Read the model definition and answer for the solid it produces. Units are mm, in the model's axes. A direction names the side the tool comes from. Coordinates: 2 decimals unless noted, no trailing zeros. Write each loop counter-clockwise with the first axis right and the second up, starting at its lowest first coordinate (ties: lowest second). Pieces come first, ordered by that corner, then holes. Notation, with made-up numbers: (43.5, 36.25) - (68.5, 36.25) arc R21 ccw to (68.5, 57.25) - close; hole circle Ø10 at (-40, -39.75). An arc over 180 degrees is marked (long way). Return JSON: item names as keys, results as strings.
```python
from build123d import *

# Parameters (mm, degrees)
SKETCH1_W           = 10
SKETCH1_H           = 4
BOSS_EXTRUDE1_DEPTH = 1
BOSS_EXTRUDE2_DEPTH = 4


with BuildPart() as part:
    # Sketch1 → Boss-Extrude1 (new body)
    with BuildSketch(Plane(origin=(0, 0, 0), x_dir=(1, 0, 0), z_dir=(0, 1, 0))):
        with BuildLine():
            Line((8.75, 22.5), (8.75, 12))
            ThreePointArc((8.75, 12), (8.530330086, 11.469669914), (8, 11.25))
            Line((8, 11.25), (0.75, 11.25))
            ThreePointArc((0.75, 11.25), (0.219669914, 11.469669914), (0, 12))
            Line((0, 12), (0, 1))
            ThreePointArc((0, 1), (0.292893219, 0.292893219), (1, 0))
            Line((1, 0), (43, 0))
            ThreePointArc((43, 0), (43.707106781, 0.292893219), (44, 1))
            Line((44, 1), (44, 33.5))
            ThreePointArc((44, 33.5), (43.707106781, 34.207106781), (43, 34.5))
            Line((43, 34.5), (1, 34.5))
            ThreePointArc((1, 34.5), (0.292893219, 34.207106781), (0, 33.5))
            Line((0, 33.5), (0, 22.5))
            ThreePointArc((0, 22.5), (0.219669914, 23.030330086), (0.75, 23.25))
            Line((0.75, 23.25), (8, 23.25))
            ThreePointArc((8, 23.25), (8.530330086, 23.030330086), (8.75, 22.5))
        make_face()
        with Locations((33, 26.5)):
            Rectangle(SKETCH1_W, SKETCH1_H, mode=Mode.SUBTRACT)
    extrude(amount=BOSS_EXTRUDE1_DEPTH)

    # Sketch1_3 → Boss-Extrude2 (add)
    with BuildSketch(Plane(origin=(0, 0, 0), x_dir=(1, 0, 0), z_dir=(0, 1, 0))):
        with BuildLine():
            ThreePointArc((43.5, 35.5), (44.560660172, 35.060660172), (45, 34))
            Line((45, 34), (45, 0.5))
            ThreePointArc((45, 0.5), (44.560660172, -0.560660172), (43.5, -1))
            Line((43.5, -1), (0.5, -1))
            ThreePointArc((0.5, -1), (-0.560660172, -0.560660172), (-1, 0.5))
            Line((-1, 0.5), (-1, 34))
            ThreePointArc((-1, 34), (-0.560660172, 35.060660172), (0.5, 35.5))
            Line((0.5, 35.5), (43.5, 35.5))
        make_face()
        with BuildLine():
            ThreePointArc((1, 34.5), (0.292893219, 34.207106781), (0, 33.5))
            Line((0, 33.5), (0, 24.75))
            Line((0, 24.75), (0, 22.5))
            Line((0, 22.5), (0, 12))
            Line((0, 12), (0, 9.75))
            Line((0, 9.75), (0, 1))
            ThreePointArc((0, 1), (0.292893219, 0.292893219), (1, 0))
            Line((1, 0), (43, 0))
            ThreePointArc((43, 0), (43.707106781, 0.292893219), (44, 1))
            Line((44, 1), (44, 33.5))
            ThreePointArc((44, 33.5), (43.707106781, 34.207106781), (43, 34.5))
            Line((43, 34.5), (1, 34.5))
        make_face(mode=Mode.SUBTRACT)
    extrude(amount=BOSS_EXTRUDE2_DEPTH)


solid = part.part
```
(1) Determine the mould class of faces 4 (the face through (45, 2, -17)), 5 (the face through (44.55, 1.97, -35.07)), 6 (the face through (43.699, 2.479, -0.285)) for opening direction Z: +Z half, -Z half, draft (parallel to the pull), parting line (faces both ways), or undercut.
Answer:
{"face 4": "draft", "face 5": "-Z half", "face 6": "undercut"}
(2) Which of the six approach directions +Z, -Z, +X, -X, +Y, -Y give full straight-line access (tool end or side, diameter ignored) to faces 1 (the face through (0, 2, -17)), 2 (the face through (32.9, 0.5, -28.5)), 3 (the face through (22, 2, 1))?
Answer:
{"face 1": "+Y", "face 2": "+Y, -Y", "face 3": "+Z, +X, -X, +Y, -Y"}
(3) A flat-ended cylindrical pin translates along its axis: P1, Ø10.5, axis at x = 28, z = -24, coming from the +Y side. Find the tip coordinate at first contact, or state that the pin passes through.
Answer:
{"P1": "y = 1"}
(4) Straight lines are drawn through the part: line 1 (Z direction, x = 3, y = 1.5); line 2 (X direction, y = 3.5, z = -4.5); line 3 (Y direction, x = 28.5, z = -31). For each, find the intervals that lie inside material, in ascending order. Write a range as from..to.
Answer:
{"line 1": "-35.5..-34.5, 0..1", "line 2": "-1..0, 44..45", "line 3": "0..1"}
(5) A cutting plane is placed at B-B (z = -18). Determine the outline of the cut face in (x, y).
Answer:
{"outline": "(-1, 0) - (0, 0) - (0, 4) - (-1, 4) - close; (8.75, 0) - (45, 0) - (45, 4) - (44, 4) - (44, 1) - (8.75, 1) - close"}
(6) A cutting plane is placed at A-A (x = 30). Determine the outline of the cut face in (y, z).
Answer:
{"outline": "(0, -35.5) - (4, -35.5) - (4, -34.5) - (1, -34.5) - (1, -28.5) - (0, -28.5) - close; (0, -24.5) - (1, -24.5) - (1, 0) - (4, 0) - (4, 1) - (0, 1) - close"}
(7) A cutting plane is placed at C-C (y = 2.7). Determine the outline of the cut face in (x, z).
Answer:
{"outline": "(-1, -34) arc R1.5 ccw to (0.5, -35.5) - (43.5, -35.5) arc R1.5 ccw to (45, -34) - (45, -0.5) arc R1.5 ccw to (43.5, 1) - (0.5, 1) arc R1.5 ccw to (-1, -0.5) - close; hole (0, -33.5) arc R1 ccw to (1, -34.5) - (43, -34.5) arc R1 ccw to (44, -33.5) - (44, -1) arc R1 ccw to (43, 0) - (1, 0) arc R1 ccw to (0, -1) - close"}
(8) A cutting plane is placed at D-D (z = -3.5). Determine the outline of the cut face in (x, y).
Answer:
{"outline": "(-1, 0) - (45, 0) - (45, 4) - (44, 4) - (44, 1) - (0, 1) - (0, 4) - (-1, 4) - close"}
